Job drawing, mm, ordinate dimensions from the low corner. One solid piece. Round coordinates to 2 decimals unless told otherwise and drop trailing zeros. Order: outer loops, then holes, each group sorted by start corner. A loop starts at its lowest first (then second) coordinate and runs counter-clockwise, first axis right, second up. Notation, with made-up numbers: M 49,89.25 L 95,89.25 A10 ccw 95,102.25 Z; hole C 25,-17 d6. An arc over 180 degrees is marked long. Answer as a JSON object with one key per item and string values. Group by question number.
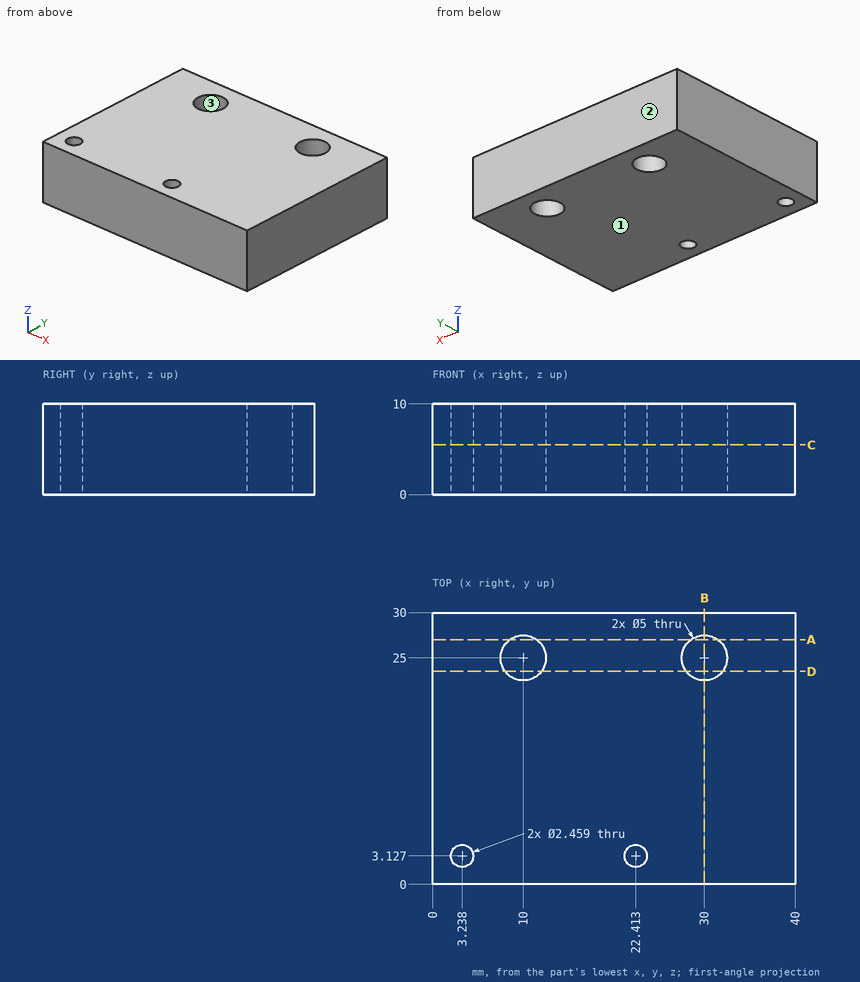
Item 1: Cut at A-A, the plane y = 27. Give the cut face in (x, z).
Item 2: Flat gauge pin, fed straight in: pin 1 Ø4 at (x, y) = (15, 10.5) entering from -Z. Where does the tip first touch, or does it go through?
Item 3: Cut at B-B, the plane x = 30. Give the cut face in (y, z).
Item 4: Drill centre lines: line 1 (X direction, y = 25, z = 9.25); line 2 (Y direction, x = 10, z = 5); line 3 (X direction, y = 3, z = 8) (1 decimal). Where is each one in solid material? Low to high. Write a range as [from, to].
Item 5: Cut at C-C, the plane z = 5.5. Give the cut face in (x, y), and give its area (3 significant figures).
Item 6: Two-plate mould, pull along Y, no slides. Class the marked faces 1, 2 and 3: +Y half, -Y half, draft (parallel to the pull), parting line (faces both ways), or undercut.
Item 7: Cut at D-D, the plane y = 23.5. Give the cut face in (x, z), and give its area (3 significant figures).
Response values:
{
 "1": {"outline": "M 0,0 L 8.5,0 L 8.5,10 L 0,10 Z; M 11.5,0 L 28.5,0 L 28.5,10 L 11.5,10 Z; M 31.5,0 L 40,0 L 40,10 L 31.5,10 Z"},
 "2": {"pin 1": "z = 0"},
 "3": {"outline": "M 0,0 L 22.5,0 L 22.5,10 L 0,10 Z; M 27.5,0 L 30,0 L 30,10 L 27.5,10 Z"},
 "4": {"line 1": "[0, 7.5], [12.5, 27.5], [32.5, 40]", "line 2": "[0, 22.5], [27.5, 30]", "line 3": "[0, 2], [4.5, 21.2], [23.6, 40]"},
 "5": {"outline": "M 0,0 L 40,0 L 40,30 L 0,30 Z; hole C 3.24,3.13 d2.46; hole C 10,25 d5; hole C 22.41,3.13 d2.46; hole C 30,25 d5", "area": "1,150 mm^2"},
 "6": {"face 1": "draft", "face 2": "+Y half", "face 3": "undercut"},
 "7": {"outline": "M 0,0 L 8,0 L 8,10 L 0,10 Z; M 12,0 L 28,0 L 28,10 L 12,10 Z; M 32,0 L 40,0 L 40,10 L 32,10 Z", "area": "320 mm^2"}
}
